Geometry: final body of the model. Coordinates: model frame, mm. A direction names the side the tool comes from. Give positions to 0.01 mm unless a question says otherwise; leave off trailing zeros. Write each loop counter-clockwise with the first axis right and the second up, starting at its lowest first coordinate (ties: lowest second). Pieces come first, ordered by that corner, then holes.
Q1. Line query: L1, parallel to X at y = 9, z = 2.5; L2, parallel to Y at x = -6, z = 2.25; L3, parallel to Y at x = -0.5, z = 2. Output: solid intervals per line, ascending.
Q2. Draft query along X for faces 1 (the face through (18.96, 11.82, 2.54)), 2 (the face through (6, 14.542, 5.7)), 3 (the face through (3.002, 7.169, 7.698)). Return one class per face: pulls with the +X half, pulls with the -X half, needs draft (parallel to the pull), parting line crosses it, or undercut.
Q3. Cut plane D-D on x = 4. Return the cut outline in (y, z), plus the area to 3 significant figures.
Q4. Reachability of faces 4 (the face through (-8.86, 11.92, 2.54)), 5 (the face through (15, 31, 5)), 6 (the face through (-5, 31, 5)) from +Z, -Z, +X, -X, +Y, -Y: full face, straight path, thin tool, end or side. Return the list, or none.
Q5. Pin query (flat end, axial travel): pin 1 (1.4 mm diameter, centred on x = 11.5, z = 2.5, fed in from +Y); pin 2 (8.5 mm diameter, centred on x = 17.5, y = 29, fed in from +Z); pin 3 (4 mm diameter, centred on y = 24.5, z = 2.5, fed in from -X). Return the tip coordinate at first contact, or that it passes through.
Q6. Cut plane A-A on x = 17.5. Return the cut outline in (y, z), plus the area to 3 significant figures.
Q7. Cut plane C-C on z = 10.75. Return the cut outline in (x, y), plus the area to 3 significant figures.
Autodesk Inventor part; units mm, degrees
ref_plane "Work Plane1" through (0, 18.542, 0) normal (0, 1, 0) x (1, 0, 0)
ref_plane "YZ Plane" through (0, 0, 0) normal (1, 0, 0) x (0, 1, 0)
ref_plane "XZ Plane" through (0, 0, 0) normal (0, 1, 0) x (-1, 0, 0)
sketch "Sketch1" plane through (0, 0, 0) normal (0, 0, 1) x (1, 0, 0)
  line L0 (0, 0) -> (10, 0)
  line L1 (10, 0) -> (10, 37.084)
  line L2 (10, 37.084) -> (0, 37.084)
  line L3 (0, 37.084) -> (0, 0)
  line L4 (0, 36.191) -> (-10.668, 36.191)
  line L5 (-10.668, 36.191) -> (-10.668, 23.491)
  line L6 (-10.668, 23.491) -> (0, 23.491)
  line L7 (0, 23.491) -> (0, 36.191)
  line L8 (0, 0.9264) -> (-10.668, 0.9264)
  line L9 (-10.668, 0.9264) -> (-10.668, 13.6264)
  line L10 (-10.668, 13.6264) -> (0, 13.6264)
  line L11 (0, 13.6264) -> (0, 0.9264)
  line L12 (5, 37.084) -> (5, 9.6109) construction
  line L13 (10, 36.191) -> (20.668, 36.191)
  line L14 (20.668, 36.191) -> (20.668, 23.491)
  line L15 (20.668, 23.491) -> (10, 23.491)
  line L16 (10, 0.9264) -> (20.668, 0.9264)
  line L17 (20.668, 0.9264) -> (20.668, 13.6264)
  line L18 (20.668, 13.6264) -> (10, 13.6264)
  line L19 (10, 36.191) -> (10, 23.491)
  line L20 (10, 13.6264) -> (10, 0.9264)
  dimension "d0" = 10
  dimension "d1" = 37.084
  dimension "d2" = 10.668
  dimension "d3" = 12.7
  dimension "d4" = 10.668
  dimension "d5" = 12.7
extrude "Extrusion1" add sketch "Sketch1" along normal blind 12.61 contours L3 L2 L1 L0
extrude "Extrusion2" add sketch "Sketch1" along normal blind 5 contours L8 L9 L10 L3 | L6 L5 L4 L3
extrude "Extrusion3" add sketch "Sketch1" along normal blind 5 contours L1 L18 L17 L16 | L1 L13 L14 L15
fillet "Fillet1" radius 5 2 edges at (10, 18.542, 12.61) (0, 18.542, 12.61)
fillet "Fillet2" radius 6 8 edges at (20.668, 36.191, 2.5) (20.668, 23.491, 2.5) (20.668, 13.6264, 2.5) (20.668, 0.9264, 2.5) (-10.668, 13.6264, 2.5) (-10.668, 36.191, 2.5) (-10.668, 23.491, 2.5) (-10.668, 0.9264, 2.5)
sketch "Sketch2" plane through (0, 0, 5) normal (0, 0, 1) x (1, 0, 0)
  arc A0 (-4.668, 13.6264) -> (-10.668, 7.6264) centre (-4.668, 7.6264) ccw
  circle A1 centre (-4.668, 7.6264) radius 1.5875
  line L0 (-4.668, 7.6264) -> (-4.668, 29.2164) construction
  line L1 (-4.668, 29.2164) -> (14.382, 29.2164) construction
  circle A2 centre (-4.668, 29.2164) radius 1.5875
  circle A3 centre (14.382, 29.2164) radius 1.5875
  circle A4 centre (14.382, 7.6264) radius 1.5875
  point P0 (0, 0)
  dimension "d14" = 3.175
  dimension "d15" = 21.59
  dimension "d16" = 19.05
  dimension "d17" = 3.175
  dimension "d18" = 3.175
  dimension "d19" = 3.175
extrude "Extrusion4" cut sketch "Sketch2" against normal blind 5
sketch "Sketch3" plane through (0, 0, 0) normal (0, -1, 0) x (1, 0, 0)
  arc A0 (10, 7.61) -> (0, 7.61) centre (5, 7.61) ccw
  circle A1 centre (5, 7.61) radius 2
  point P0 (0, 0)
  dimension "d22" = 4
extrude "Extrusion5" cut sketch "Sketch3" against normal blind 100
ref_plane "Work Plane1" through (0, 18.542, 0) normal (0, 1, 0) x (1, 0, 0)
sketch "Sketch4" plane through (0, 18.542, 0) normal (0, 1, 0) x (1, 0, 0)
  arc A0 (0, -7.61) -> (10, -7.61) centre (5, -7.61) ccw construction
  line L0 (5, -12.61) -> (5, -1.47) construction
  line L1 (10, -1.47) -> (0, -1.47)
  line L2 (0, 0) -> (0, -7.61)
  line L3 (0, -1.47) -> (-2.5969, -14.0453)
  line L4 (-2.5969, -14.0453) -> (12.3635, -14.2385)
  line L5 (12.3635, -14.2385) -> (10, -1.47)
  dimension "d25" = 11.14
extrude "Extrusion6" cut sketch "Sketch4" along normal mid plane 8
properties part number "Nose Gear Mounting Block"
Data:
1. L1: x = -10.51 to -5.46, -3.87 to 13.59, 15.18 to 20.51
1. L2: y = 1.08 to 6.76, 8.49 to 13.48, 23.64 to 28.35, 30.08 to 36.04
1. L3: y = 0.93 to 13.63, 23.49 to 36.19
2. face 1: pulls with the +X half
2. face 2: needs draft
2. face 3: undercut
3. outline: (0, 0) - (37.08, 0) - (37.08, 5.88) - (22.54, 5.88) - (22.54, 1.47) - (14.54, 1.47) - (14.54, 5.88) - (0, 5.88) - close; (0, 9.34) - (14.54, 9.34) - (14.54, 12.51) - (0, 12.51) - close; (22.54, 9.34) - (37.08, 9.34) - (37.08, 12.51) - (22.54, 12.51) - close
3. area: 275 mm2
4. face 4: +Z, -Z, -X
4. face 5: +Z, +X, +Y, -Y
4. face 6: +Z, -X, +Y, -Y
5. pin 1: stops at y = 36.19
5. pin 2: stops at z = 5
5. pin 3: stops at x = -9.87
6. outline: (1.64, 0) - (12.92, 0) - (12.92, 5) - (1.64, 5) - close; (24.2, 0) - (35.48, 0) - (35.48, 5) - (24.2, 5) - close
6. area: 113 mm2
7. outline: (1.11, 0) - (8.89, 0) - (8.89, 14.54) - (1.11, 14.54) - close; (1.11, 22.54) - (8.89, 22.54) - (8.89, 37.08) - (1.11, 37.08) - close
7. area: 226 mm2
